from build123d import *

# Parameters (mm, degrees)
BOSS_EXTRUDE1_DEPTH = 50.8
SKETCH2_W           = 12.7
SKETCH2_H           = 3.175
CUT_EXTRUDE1_DEPTH  = 3.175


with BuildPart() as part:
    # Sketch1 → Boss-Extrude1 (new body)
    with BuildSketch(Plane.XY):
        Polygon((39.563966172, 294.491722579), (40.233488411, 291.388117421), (71.269539981, 298.083339818), (70.600017742, 301.186944975), align=None)
    extrude(amount=-BOSS_EXTRUDE1_DEPTH)

    # Sketch2 → Cut-Extrude1 (cut)
    with BuildSketch(Plane(origin=(-58.944661512, 273.241043546, 0), x_dir=(0.977513435, 0.210873146, 0), z_dir=(-0.210873146, 0.977513435, 0))):
        with Locations((116.649704601, 49.2125)):
            Rectangle(SKETCH2_W, SKETCH2_H)
        with Locations((116.649704601, 1.5875)):
            Rectangle(SKETCH2_W, SKETCH2_H)
    extrude(amount=-CUT_EXTRUDE1_DEPTH, mode=Mode.SUBTRACT)


solid = part.part
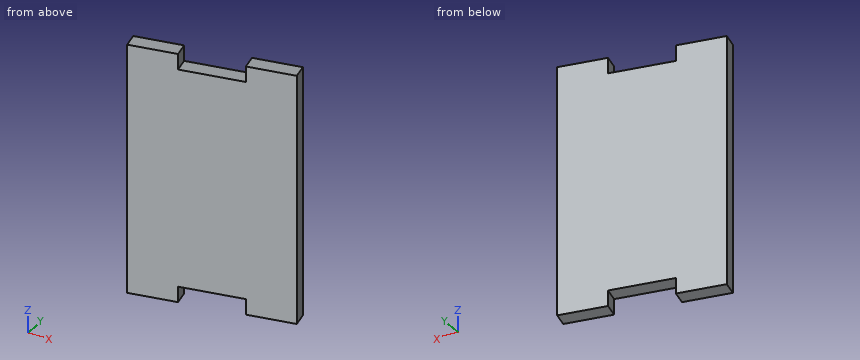
Design review of the part built by this model. Coordinates are the model's own, in mm. Coordinates: 2 decimals unless noted, no trailing zeros. Order: outer loops, then holes, each group sorted by start corner. A loop starts at its lowest first (then second) coordinate and runs counter-clockwise, first axis right, second up. Notation, with made-up numbers: M 76,-8 L 100,-8 A16 cw 100,22 Z; hole C -3.5,22 d6. An arc over 180 degrees is marked long. Use a Markdown table: item, result.
(1) Add section B-B (z = -14). Give the boundary of the cut face in (x, y).
Worked answers:
| item | result |
|---|---|
| outline | M 39.56,294.49 L 40.23,291.39 L 71.27,298.08 L 70.6,301.19 Z |
(2) Wall thickness on probe 1 along Z at (x, y) = (50.5, 295) (3 decimals); probe 2 along Y at (x, z) = (49.5, -22); probe 3 along Y at (x, z) = (60, -20): over which ranges is each line inside the solid? List them lowest first.
Worked answers:
| item | result |
|---|---|
| probe 1 | z = -47.625 to -3.175 |
| probe 2 | y = 293.39 to 296.64 |
| probe 3 | y = 295.65 to 298.9 |
(3) Add section A-A (y = 297). Give the boundary of the cut face in (x, z) (3 decimals).
Worked answers:
| item | result |
|---|---|
| outline | M 51.191,-47.625 L 61.759,-47.625 L 61.759,-50.8 L 66.248,-50.8 L 66.248,0 L 61.759,0 L 61.759,-3.175 L 51.191,-3.175 Z |
(4) Add section C-C (x = 55.5). Give the boundary of the cut face in (y, z) (1 decimal), then the cut area to 3 significant figures.
Worked answers:
| item | result |
|---|---|
| outline | M 294.7,-47.6 L 297.9,-47.6 L 297.9,-3.2 L 294.7,-3.2 Z |
| area | 144 mm2 |
(5) For P1, Ø5, axis at x = 53, z = -43.5, coming from the +Y side; P2, Ø6, axis at x = 43, z = -35, coming from the -Y side; P3, Ø4, axis at y = 299, z = -39.5, coming from the +X side, all flat-tipped, find the tip position at first contact; note any pin that passes through.
Worked answers:
| item | result |
|---|---|
| P1 | stops at y = 297.93 |
| P2 | stops at y = 291.39 |
| P3 | stops at x = 71.27 |
